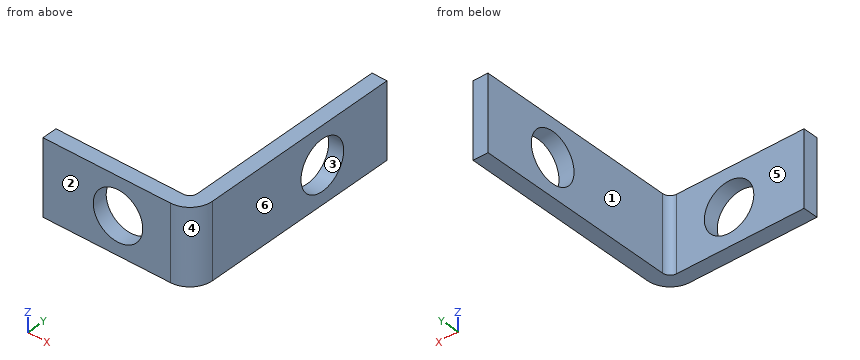
from build123d import *

# Parameters (mm, degrees)
BRIDA_BASE1_DEPTH                          = 5
TALADRO_DE_MARGEN_PARA_M65_D               = 6.6
TALADRO_DE_MARGEN_PARA_M65_DEPTH           = 11.62
TALADRO_DE_MARGEN_PARA_M65_TIP             = 1.982840043
TALADRO_DE_MARGEN_PARA_M65_ON_FACE_2_D     = 6.6
TALADRO_DE_MARGEN_PARA_M65_ON_FACE_2_DEPTH = 11.62
TALADRO_DE_MARGEN_PARA_M65_ON_FACE_2_TIP   = 1.982840043


# Sheet-metal steps are written as plain solids
with BuildPart() as part:
    # Croquis1 → Brida base1 (new, symmetric)
    with BuildSketch(Plane.XY):
        with BuildLine():
            Line((0, 30), (0, 3))
            ThreePointArc((0, 3), (-0.878679656, 0.878679656), (-3, 0))
            Line((-3, 0), (-20, 0))
            Line((-20, 0), (-20, 2))
            Line((-20, 2), (-3, 2))
            ThreePointArc((-3, 2), (-2.292893219, 2.292893219), (-2, 3))
            Line((-2, 3), (-2, 30))
            Line((-2, 30), (0, 30))
        make_face()
    extrude(amount=BRIDA_BASE1_DEPTH, both=True)

    # Taladro de margen para M65
    with Locations(Plane(origin=(0, 20, 0), x_dir=(0, 1, 0), z_dir=(1, 0, 0))):
        with Locations((0, 0)):
            Hole(TALADRO_DE_MARGEN_PARA_M65_D / 2, depth=TALADRO_DE_MARGEN_PARA_M65_DEPTH)
            with Locations((0, 0, -(TALADRO_DE_MARGEN_PARA_M65_DEPTH + TALADRO_DE_MARGEN_PARA_M65_TIP / 2))):  # 118° drill point
                Cone(0, TALADRO_DE_MARGEN_PARA_M65_D / 2, TALADRO_DE_MARGEN_PARA_M65_TIP, mode=Mode.SUBTRACT)

    # Taladro de margen para M65 on face 2
    with Locations(Plane(origin=(-10, 2, 0), x_dir=(0, 0, 1), z_dir=(0, 1, 0))):
        with Locations((0, 0)):
            Hole(TALADRO_DE_MARGEN_PARA_M65_ON_FACE_2_D / 2, depth=TALADRO_DE_MARGEN_PARA_M65_ON_FACE_2_DEPTH)
            with Locations((0, 0, -(TALADRO_DE_MARGEN_PARA_M65_ON_FACE_2_DEPTH + TALADRO_DE_MARGEN_PARA_M65_ON_FACE_2_TIP / 2))):  # 118° drill point
                Cone(0, TALADRO_DE_MARGEN_PARA_M65_ON_FACE_2_D / 2, TALADRO_DE_MARGEN_PARA_M65_ON_FACE_2_TIP, mode=Mode.SUBTRACT)


solid = part.part
Here's how the part is built. I have some questions about the finished solid (model axes, mm). Face numbers are marked on the shaded views. A direction names the side the tool comes from. Coordinates: 2 decimals unless noted, no trailing zeros. Write each loop counter-clockwise with the first axis right and the second up, starting at its lowest first coordinate (ties: lowest second). Pieces come first, ordered by that corner, then holes.
Item 1: On a 3-axis mill with a long thin cutter (end or side, diameter ignored), from which of +Z, -Z, +X, -X, +Y, -Y can I reach the whole of each face in a straight line? I mean the marked faces 1 and 2. Say none if no direction works.
Item 2: If we mould it in two halves opening along Y, with no side actions, what happens to the marked faces 3, 4, 5 and 6? For each: +Y half, -Y half, draft (parallel to the pull), parting line (faces both ways), or undercut.
Item 3: If I drill on line 1 (Y direction, x = -14.5, z = 1.5); line 2 (Z direction, x = -1.4, y = 20); line 3 (X direction, y = 11.25, z = -0.5), over which ranges is the centre line in solid material (lowest first)?
Item 4: I want a section at A-A on y = 20. Write out the boundary of the cut face in (x, z).
Item 5: Will these pins go through, and if not, where does the flat tip stop? pin 1 (1.5 mm diameter, centred on y = 7, z = -3.5, fed in from +X); pin 2 (5 mm diameter, centred on y = 20.5, z = -2, fed in from -X); pin 3 (1 mm diameter, centred on x = -15.5, z = 0, fed in from +Y).
Item 6: I want a section at B-B on z = 0. Write out the boundary of the cut face in (x, y), and give its area (3 significant figures).
Item 7: I want a section at C-C on x = -10. Write out the boundary of the cut face in (y, z).
Item 8: I want a section at D-D on z = 1.5. Write out the boundary of the cut face in (x, y).
Findings below:
1. face 1: +Z, -Z, -X, +Y
1. face 2: +Z, -Z, +X, -X, -Y
2. face 3: undercut
2. face 4: -Y half
2. face 5: +Y half
2. face 6: draft
3. line 1: y = 0 to 2
3. line 2: z = -5 to -3.3, 3.3 to 5
3. line 3: x = -2 to 0
4. outline: (-2, -5) - (0, -5) - (0, -3.3) - (-2, -3.3) - close; (-2, 3.3) - (0, 3.3) - (0, 5) - (-2, 5) - close
5. pin 1: stops at x = 0
5. pin 2: stops at x = -2
5. pin 3: stops at y = 2
6. outline: (-20, 0) - (-13.3, 0) - (-13.3, 2) - (-20, 2) - close; (-6.7, 0) - (-3, 0) arc R3 ccw to (0, 3) - (0, 16.7) - (-2, 16.7) - (-2, 3) arc R1 cw to (-3, 2) - (-6.7, 2) - close; (-2, 23.3) - (0, 23.3) - (0, 30) - (-2, 30) - close
6. area: 67.9 mm2
7. outline: (0, -5) - (2, -5) - (2, -3.3) - (0, -3.3) - close; (0, 3.3) - (2, 3.3) - (2, 5) - (0, 5) - close
8. outline: (-20, 0) - (-12.94, 0) - (-12.94, 2) - (-20, 2) - close; (-7.06, 0) - (-3, 0) arc R3 ccw to (0, 3) - (0, 17.06) - (-2, 17.06) - (-2, 3) arc R1 cw to (-3, 2) - (-7.06, 2) - close; (-2, 22.94) - (0, 22.94) - (0, 30) - (-2, 30) - close
